Read the model definition and answer for the solid it produces. Units are mm, in the model's axes. A direction names the side the tool comes from. Give positions to 0.01 mm unless a question says otherwise; leave off trailing zeros. Order: outer loops, then holes, each group sorted by start corner. A loop starts at its lowest first (then second) coordinate and runs counter-clockwise, first axis right, second up. Notation, with made-up numbers: (41, -31.75) -> (71, -31.75) arc R26 ccw to (71, -12.75) -> close; hole circle Ø1 at (-28, -26). An arc over 180 degrees is marked (long way). Answer as CSV lines item,"result". Start each with the question number.
1) For faces 1 (the face through (-0.149, 8.355, 1.565)), 2 (the face through (-12, 0, 52.965)), determine the directions among +Z, -Z, +X, -X, +Y, -Y from which every point of the face is accessible in a straight line to the end or side of a thin tool.
2) Find section B-B (y = -12). Determine the outline of the cut face in (x, z) (3 decimals), and give its area (3 significant figures).
3) Flat-ended cylindrical pins translate along their axes: pin 1 Ø2.5 at (x, y) = (-5.43, 5.34) entering from +Z (3 decimals); pin 2 Ø3 at (x, z) = (-11.5, 27) entering from -Y (3 decimals); pin 3 Ø7 at (x, z) = (-12.5, 42.5) entering from +Y (3 decimals); pin 4 Ø1.2 at (x, y) = (-6.52, 2.55) entering from +Z. Find the tip coordinate at first contact, or state that the pin passes through.
4) Find section A-A (z = 34). Determine the outline of the cut face in (x, y) (3 decimals), and give its area (3 significant figures).
5) The mould has two halves that part along X. Classify faces 3 (the face through (3, 0, 3.175)), 4 (the face through (-15.964, -0.218, 3.939)), 5 (the face through (0.409, -8.344, 1.565)): +X half, -X half, draft (parallel to the pull), parting line (faces both ways), or undercut.
6) Find section C-C (x = 11). Determine the outline of the cut face in (y, z) (3 decimals).
7) Straight lines are drawn through the part: L1, parallel to Z at x = -10.5, y = 0.5 (3 decimals); L2, parallel to X at y = 13, z = 56.5; L3, parallel to Z at x = -4.5, y = 3 (3 decimals). For each, find the intervals that lie inside material, in ascending order. Write a range as from..to.
8) Find section D-D (y = 20). Determine the outline of the cut face in (x, z) (3 decimals), and give its area (3 significant figures).
```python
from build123d import *

# Parameters (mm, degrees)
SKETCH1_R           = 23.495
BOSS_EXTRUDE1_DEPTH = 3.175
SKETCH4_W           = 58.68
SKETCH4_H           = 26.35
SKETCH4_R           = 2
SKETCH4_W_2         = 40.9
SKETCH4_H_2         = 20
BOSS_EXTRUDE3_DEPTH = 6.35
FILLET1_R           = 2.54
CUT_EXTRUDE1_REACH  = 72.214
SKETCH5_R           = 0.75
SKETCH5_R_2         = 1.5
SKETCH6_R           = 2.2
CUT_EXTRUDE2_DEPTH  = 68.434208377
FILLET2_R           = 2.54


with BuildPart() as part:
    # Sketch1 → Boss-Extrude1 (new body)
    with BuildSketch(Plane.XY):
        Circle(SKETCH1_R)
    extrude(amount=BOSS_EXTRUDE1_DEPTH)

    # Sketch4 → Boss-Extrude3 (add)
    with BuildSketch(Plane(origin=(-8.89, 0, 0), x_dir=(0, 0, -1), z_dir=(1, 0, 0))):
        with Locations((-32.515, 0)):
            Rectangle(SKETCH4_W, SKETCH4_H)
        with Locations((-56.815, -5)):
            Circle(SKETCH4_R, mode=Mode.SUBTRACT)
        with Locations((-56.815, 5)):
            Circle(SKETCH4_R, mode=Mode.SUBTRACT)
        with Locations((-8.215, -5)):
            Circle(SKETCH4_R, mode=Mode.SUBTRACT)
        with Locations((-8.215, 5)):
            Circle(SKETCH4_R, mode=Mode.SUBTRACT)
        with Locations((-32.515, 0)):
            Rectangle(SKETCH4_W_2, SKETCH4_H_2, mode=Mode.SUBTRACT)
    extrude(amount=-BOSS_EXTRUDE3_DEPTH)

    # Fillet1
    # the kernel refuses this fillet: 2.54 mm, written as the material it adds along each edge
    with BuildSketch(Plane(origin=(-15.24, -13.175, 3.175), x_dir=(-1, 0, 0), z_dir=(0, 1, 0))) as fillet1_piece_1:
        with BuildLine():
            CenterArc((FILLET1_R, FILLET1_R), FILLET1_R, 180, 90)
            Line((0, FILLET1_R), (0, 0))
            Line((0, 0), (FILLET1_R, 0))
        make_face()
    extrude(amount=26.35)
    with BuildSketch(Plane(origin=(-8.89, 13.175, 3.175), x_dir=(0, 1, 0), z_dir=(-1, 0, 0))) as fillet1_piece_2:
        with BuildLine():
            CenterArc((FILLET1_R, -FILLET1_R), FILLET1_R, 90, 90)
            Line((0, -FILLET1_R), (0, 0))
            Line((0, 0), (FILLET1_R, 0))
        make_face()
    extrude(amount=6.35)
    with BuildSketch(Plane(origin=(-8.89, -13.175, 3.175), x_dir=(0, -1, 0), z_dir=(-1, 0, 0))) as fillet1_piece_3:
        with BuildLine():
            CenterArc((FILLET1_R, FILLET1_R), FILLET1_R, 180, 90)
            Line((0, FILLET1_R), (0, 0))
            Line((0, 0), (FILLET1_R, 0))
        make_face()
    extrude(amount=6.35)
    with BuildSketch(Plane(origin=(-15.24, -19.525, 3.175), x_dir=(-1, 0, 0), z_dir=(0, 1, 0))) as fillet1_piece_4a_section:
        with BuildLine():
            CenterArc((FILLET1_R, FILLET1_R), FILLET1_R, 180, 90)
            Line((0, FILLET1_R), (0, 0))
            Line((0, 0), (FILLET1_R, 0))
        make_face()
    fillet1_piece_4a = extrude(amount=32.7, mode=Mode.PRIVATE)
    fillet1_piece_4a = fillet1_piece_4a & Plane(origin=(0, 0, 3.789458471), x_dir=(1, 0, 0), z_dir=(0, 0, -1)) * Cylinder(23.495, 76, mode=Mode.PRIVATE)
    fillet1_piece_4a = split(fillet1_piece_4a, bisect_by=Plane(origin=(-15.747234341, -13.175, 3.789458471), z_dir=(0, -1, 0)), keep=Keep.TOP, mode=Mode.PRIVATE)
    with BuildSketch(Plane(origin=(-8.89, -13.175, 3.175), x_dir=(0, -1, 0), z_dir=(-1, 0, 0))) as fillet1_piece_4b_section:
        with BuildLine():
            CenterArc((FILLET1_R, FILLET1_R), FILLET1_R, 180, 90)
            Line((0, FILLET1_R), (0, 0))
            Line((0, 0), (FILLET1_R, 0))
        make_face()
    fillet1_piece_4b = extrude(amount=12.7, mode=Mode.PRIVATE)
    fillet1_piece_4b = fillet1_piece_4b & Plane(origin=(0, 0, 3.784403855), x_dir=(1, 0, 0), z_dir=(0, 0, -1)) * Cylinder(23.495, 36, mode=Mode.PRIVATE)
    fillet1_piece_4b = split(fillet1_piece_4b, bisect_by=Plane(origin=(-15.24, -13.690986617, 3.784403855), z_dir=(-1, 0, 0)), keep=Keep.TOP, mode=Mode.PRIVATE)
    fillet1_piece_4 = fillet1_piece_4a & fillet1_piece_4b
    add(fillet1_piece_4)
    with BuildSketch(Plane(origin=(-8.89, 13.175, 3.175), x_dir=(0, 1, 0), z_dir=(-1, 0, 0))) as fillet1_piece_5a_section:
        with BuildLine():
            CenterArc((FILLET1_R, -FILLET1_R), FILLET1_R, 90, 90)
            Line((0, -FILLET1_R), (0, 0))
            Line((0, 0), (FILLET1_R, 0))
        make_face()
    fillet1_piece_5a = extrude(amount=12.7, mode=Mode.PRIVATE)
    fillet1_piece_5a = fillet1_piece_5a & Plane(origin=(0, 0, 3.784403835), x_dir=(1, 0, 0), z_dir=(0, 0, -1)) * Cylinder(23.495, 36, mode=Mode.PRIVATE)
    fillet1_piece_5a = split(fillet1_piece_5a, bisect_by=Plane(origin=(-15.24, 13.69098675, 3.784403835), z_dir=(-1, 0, 0)), keep=Keep.TOP, mode=Mode.PRIVATE)
    with BuildSketch(Plane(origin=(-15.24, -13.175, 3.175), x_dir=(-1, 0, 0), z_dir=(0, 1, 0))) as fillet1_piece_5b_section:
        with BuildLine():
            CenterArc((FILLET1_R, FILLET1_R), FILLET1_R, 180, 90)
            Line((0, FILLET1_R), (0, 0))
            Line((0, 0), (FILLET1_R, 0))
        make_face()
    fillet1_piece_5b = extrude(amount=32.7, mode=Mode.PRIVATE)
    fillet1_piece_5b = fillet1_piece_5b & Plane(origin=(0, 0, 3.789458493), x_dir=(1, 0, 0), z_dir=(0, 0, -1)) * Cylinder(23.495, 76, mode=Mode.PRIVATE)
    fillet1_piece_5b = split(fillet1_piece_5b, bisect_by=Plane(origin=(-15.747234214, 13.175, 3.789458493), z_dir=(0, 1, 0)), keep=Keep.TOP, mode=Mode.PRIVATE)
    fillet1_piece_5 = fillet1_piece_5a & fillet1_piece_5b
    add(fillet1_piece_5)

    # Sketch5 → Cut-Extrude1 (cut, up to next)
    with BuildSketch(Plane(origin=(0, 0, 0), x_dir=(-1, 0, 0), z_dir=(0, 0, -1)), mode=Mode.PRIVATE) as cut_extrude1_sk1:
        with Locations((5.342004985, -5.427981461)):
            Circle(SKETCH5_R)
    cut_extrude1_tool1 = extrude(cut_extrude1_sk1.sketch, amount=-CUT_EXTRUDE1_REACH, mode=Mode.PRIVATE) & part.part
    # Sketch5 → Cut-Extrude1 (cut, up to next)
    with BuildSketch(Plane(origin=(0, 0, 0), x_dir=(-1, 0, 0), z_dir=(0, 0, -1)), mode=Mode.PRIVATE) as cut_extrude1_sk2:
        with Locations((2.547769545, -6.519882694)):
            Circle(SKETCH5_R)
    cut_extrude1_tool2 = extrude(cut_extrude1_sk2.sketch, amount=-CUT_EXTRUDE1_REACH, mode=Mode.PRIVATE) & part.part
    # Sketch5 → Cut-Extrude1 (cut, up to next)
    with BuildSketch(Plane(origin=(0, 0, 0), x_dir=(-1, 0, 0), z_dir=(0, 0, -1)), mode=Mode.PRIVATE) as cut_extrude1_sk3:
        with Locations((-0.246465895, -7.611783928)):
            Circle(SKETCH5_R)
    cut_extrude1_tool3 = extrude(cut_extrude1_sk3.sketch, amount=-CUT_EXTRUDE1_REACH, mode=Mode.PRIVATE) & part.part
    # Sketch5 → Cut-Extrude1 (cut, up to next)
    with BuildSketch(Plane(origin=(0, 0, 0), x_dir=(-1, 0, 0), z_dir=(0, 0, -1)), mode=Mode.PRIVATE) as cut_extrude1_sk4:
        with Locations((-5.427981461, -5.342004985)):
            Circle(SKETCH5_R)
    cut_extrude1_tool4 = extrude(cut_extrude1_sk4.sketch, amount=-CUT_EXTRUDE1_REACH, mode=Mode.PRIVATE) & part.part
    # Sketch5 → Cut-Extrude1 (cut, up to next)
    with BuildSketch(Plane(origin=(0, 0, 0), x_dir=(-1, 0, 0), z_dir=(0, 0, -1)), mode=Mode.PRIVATE) as cut_extrude1_sk5:
        with Locations((-6.519882694, -2.547769545)):
            Circle(SKETCH5_R)
    cut_extrude1_tool5 = extrude(cut_extrude1_sk5.sketch, amount=-CUT_EXTRUDE1_REACH, mode=Mode.PRIVATE) & part.part
    # Sketch5 → Cut-Extrude1 (cut, up to next)
    with BuildSketch(Plane(origin=(0, 0, 0), x_dir=(-1, 0, 0), z_dir=(0, 0, -1)), mode=Mode.PRIVATE) as cut_extrude1_sk6:
        with Locations((-7.611783928, 0.246465895)):
            Circle(SKETCH5_R)
    cut_extrude1_tool6 = extrude(cut_extrude1_sk6.sketch, amount=-CUT_EXTRUDE1_REACH, mode=Mode.PRIVATE) & part.part
    # Sketch5 → Cut-Extrude1 (cut, up to next)
    with BuildSketch(Plane(origin=(0, 0, 0), x_dir=(-1, 0, 0), z_dir=(0, 0, -1)), mode=Mode.PRIVATE) as cut_extrude1_sk7:
        with Locations((-5.342004985, 5.427981461)):
            Circle(SKETCH5_R)
    cut_extrude1_tool7 = extrude(cut_extrude1_sk7.sketch, amount=-CUT_EXTRUDE1_REACH, mode=Mode.PRIVATE) & part.part
    # Sketch5 → Cut-Extrude1 (cut, up to next)
    with BuildSketch(Plane(origin=(0, 0, 0), x_dir=(-1, 0, 0), z_dir=(0, 0, -1)), mode=Mode.PRIVATE) as cut_extrude1_sk8:
        with Locations((-2.547769545, 6.519882694)):
            Circle(SKETCH5_R)
    cut_extrude1_tool8 = extrude(cut_extrude1_sk8.sketch, amount=-CUT_EXTRUDE1_REACH, mode=Mode.PRIVATE) & part.part
    # Sketch5 → Cut-Extrude1 (cut, up to next)
    with BuildSketch(Plane(origin=(0, 0, 0), x_dir=(-1, 0, 0), z_dir=(0, 0, -1)), mode=Mode.PRIVATE) as cut_extrude1_sk9:
        with Locations((0.246465895, 7.611783928)):
            Circle(SKETCH5_R)
    cut_extrude1_tool9 = extrude(cut_extrude1_sk9.sketch, amount=-CUT_EXTRUDE1_REACH, mode=Mode.PRIVATE) & part.part
    # Sketch5 → Cut-Extrude1 (cut, up to next)
    with BuildSketch(Plane(origin=(0, 0, 0), x_dir=(-1, 0, 0), z_dir=(0, 0, -1)), mode=Mode.PRIVATE) as cut_extrude1_sk10:
        with Locations((5.427981461, 5.342004985)):
            Circle(SKETCH5_R)
    cut_extrude1_tool10 = extrude(cut_extrude1_sk10.sketch, amount=-CUT_EXTRUDE1_REACH, mode=Mode.PRIVATE) & part.part
    # Sketch5 → Cut-Extrude1 (cut, up to next)
    with BuildSketch(Plane(origin=(0, 0, 0), x_dir=(-1, 0, 0), z_dir=(0, 0, -1)), mode=Mode.PRIVATE) as cut_extrude1_sk11:
        with Locations((6.519882694, 2.547769545)):
            Circle(SKETCH5_R)
    cut_extrude1_tool11 = extrude(cut_extrude1_sk11.sketch, amount=-CUT_EXTRUDE1_REACH, mode=Mode.PRIVATE) & part.part
    # Sketch5 → Cut-Extrude1 (cut, up to next)
    with BuildSketch(Plane(origin=(0, 0, 0), x_dir=(-1, 0, 0), z_dir=(0, 0, -1)), mode=Mode.PRIVATE) as cut_extrude1_sk12:
        with Locations((7.611783928, -0.246465895)):
            Circle(SKETCH5_R)
    cut_extrude1_tool12 = extrude(cut_extrude1_sk12.sketch, amount=-CUT_EXTRUDE1_REACH, mode=Mode.PRIVATE) & part.part
    # Sketch5 → Cut-Extrude1 (cut, up to next)
    with BuildSketch(Plane(origin=(0, 0, 0), x_dir=(-1, 0, 0), z_dir=(0, 0, -1)), mode=Mode.PRIVATE) as cut_extrude1_sk13:
        Circle(SKETCH5_R_2)
    cut_extrude1_tool13 = extrude(cut_extrude1_sk13.sketch, amount=-CUT_EXTRUDE1_REACH, mode=Mode.PRIVATE) & part.part
    add(cut_extrude1_tool1.solids().sort_by_distance((-5.342005, -5.427981, 0))[0], mode=Mode.SUBTRACT)
    add(cut_extrude1_tool2.solids().sort_by_distance((-2.54777, -6.519883, 0))[0], mode=Mode.SUBTRACT)
    add(cut_extrude1_tool3.solids().sort_by_distance((0.246466, -7.611784, 0))[0], mode=Mode.SUBTRACT)
    add(cut_extrude1_tool4.solids().sort_by_distance((5.427981, -5.342005, 0))[0], mode=Mode.SUBTRACT)
    add(cut_extrude1_tool5.solids().sort_by_distance((6.519883, -2.54777, 0))[0], mode=Mode.SUBTRACT)
    add(cut_extrude1_tool6.solids().sort_by_distance((7.611784, 0.246466, 0))[0], mode=Mode.SUBTRACT)
    add(cut_extrude1_tool7.solids().sort_by_distance((5.342005, 5.427981, 0))[0], mode=Mode.SUBTRACT)
    add(cut_extrude1_tool8.solids().sort_by_distance((2.54777, 6.519883, 0))[0], mode=Mode.SUBTRACT)
    add(cut_extrude1_tool9.solids().sort_by_distance((-0.246466, 7.611784, 0))[0], mode=Mode.SUBTRACT)
    add(cut_extrude1_tool10.solids().sort_by_distance((-5.427981, 5.342005, 0))[0], mode=Mode.SUBTRACT)
    add(cut_extrude1_tool11.solids().sort_by_distance((-6.519883, 2.54777, 0))[0], mode=Mode.SUBTRACT)
    add(cut_extrude1_tool12.solids().sort_by_distance((-7.611784, -0.246466, 0))[0], mode=Mode.SUBTRACT)
    add(cut_extrude1_tool13.solids().sort_by_distance((0, 0, 0))[0], mode=Mode.SUBTRACT)

    # Sketch6 → Cut-Extrude2 (cut, through all)
    with BuildSketch(Plane.XY.offset(3.175)):
        Circle(SKETCH6_R)
    extrude(amount=-CUT_EXTRUDE2_DEPTH, mode=Mode.SUBTRACT)

    # Fillet2
    fillet2_edges = [part.edges().sort_by_distance(p)[0] for p in [
        (-12.065, -13.175, 61.855),
        (-12.065, 13.175, 61.855),
    ]]
    fillet(fillet2_edges, radius=FILLET2_R)


solid = part.part
```
Findings below:
1,face 1,"+Z, -Z"
1,face 2,"+X, -X"
2,outline,"(-20.199, 0) -> (20.199, 0) -> (20.199, 3.175) -> (-8.89, 3.175) -> (-8.89, 61.457) -> (-15.24, 61.457) -> (-15.24, 5.715) arc R2.54 cw to (-17.78, 3.175) -> (-20.199, 3.175) -> close"
2,area,"500 mm²"
3,pin 1,"z = 3.175"
3,pin 2,"y = -13.175"
3,pin 3,"y = 13.175"
3,pin 4,"through"
4,outline,"(-15.24, -13.175) -> (-8.89, -13.175) -> (-8.89, -10) -> (-15.24, -10) -> close; (-15.24, 10) -> (-8.89, 10) -> (-8.89, 13.175) -> (-15.24, 13.175) -> close"
4,area,"40.3 mm²"
5,face 3,"draft"
5,face 4,"-X half"
5,face 5,"undercut"
6,outline,"(-20.761, 0) -> (20.761, 0) -> (20.761, 3.175) -> (-20.761, 3.175) -> close"
7,L1,"0..12.065, 52.965..61.855"
7,L2,"-15.24..-8.89"
7,L3,"0..3.175"
8,outline,"(-12.329, 0) -> (12.329, 0) -> (12.329, 3.175) -> (-12.329, 3.175) -> close"
8,area,"78.3 mm²"
